Can you work these out from the model? Positions are in its coordinate system, mm. Face numbers are marked on the shaded views. A direction names the side the tool comes from. Give positions to 0.01 mm unless a question says otherwise; leave off trailing zeros. Loops run counter-clockwise (first coordinate to the right, second up) from the corner with the lowest first, then second, coordinate; pieces in that order, holes last.
Autodesk Inventor part; units mm, degrees
ref_plane "YZ Plane" through (0, 0, 0) normal (1, 0, 0) x (0, 1, 0)
ref_plane "XZ Plane" through (0, 0, 0) normal (0, 1, 0) x (-1, 0, 0)
ref_plane "XY Plane" through (0, 0, 0) normal (0, 0, 1) x (1, 0, 0)
sketch "Sketch1" plane through (0, 0, 0) normal (0, 1, 0) x (-1, 0, 0)
  line L0 (-48.611, 110.4452) -> (-48.611, 10.4452)
  line L1 (-48.611, 111.4452) -> (52.389, 111.4452)
  line L2 (52.389, 111.4452) -> (52.389, 9.4452)
  line L3 (52.389, 9.4452) -> (-48.611, 9.4452)
  line L4 (-48.611, 10.4452) -> (-48.611, 9.4452)
  line L5 (-48.611, 110.4452) -> (-48.611, 111.4452)
  line L6 (54.389, 7.4452) -> (54.389, 113.4452)
  line L7 (54.389, 113.4452) -> (-50.611, 113.4452)
  line L8 (-50.611, 113.4452) -> (-50.611, 110.4452)
  line L9 (-50.611, 110.4452) -> (-50.611, 10.4452)
  line L10 (-50.611, 10.4452) -> (-50.611, 7.4452)
  line L11 (-50.611, 7.4452) -> (54.389, 7.4452)
  point P0 (0, 0)
  dimension "d1" = 2
extrude "Extrusion1" add sketch "Sketch1" along normal blind 25
sketch "Sketch2" plane through (0, 25, 0) normal (0, 1, 0) x (1, 0, 0)
  line L0 (-54.389, -7.4452) -> (-54.389, -113.4452)
  line L1 (50.611, -113.4452) -> (50.611, -7.4452)
  line L2 (-54.389, -113.4452) -> (50.611, -113.4452)
  line L3 (50.611, -113.4452) -> (50.611, -7.4452)
  line L4 (50.611, -7.4452) -> (-54.389, -7.4452)
  line L5 (-54.389, -7.4452) -> (-54.389, -113.4452)
  point P0 (0, 0)
extrude "Extrusion2" add sketch "Sketch2" along normal blind 2
sketch "Sketch3" plane through (0, 25, 0) normal (0, -1, 0) x (1, 0, 0)
  line L0 (48.611, 9.4452) -> (48.611, 111.4452)
  line L1 (48.611, 111.4452) -> (-52.389, 111.4452)
  line L2 (-52.389, 111.4452) -> (-52.389, 9.4452)
  line L3 (-52.389, 9.4452) -> (48.611, 9.4452)
  line L4 (-52.389, 9.4452) -> (-43.389, 9.4452)
  line L5 (-43.389, 9.4452) -> (-43.389, 18.4452)
  line L6 (-43.389, 18.4452) -> (-52.389, 18.4452)
  line L7 (-52.389, 18.4452) -> (-52.389, 9.4452)
  line L8 (48.611, 9.4452) -> (39.611, 9.4452)
  line L9 (39.611, 9.4452) -> (39.611, 18.4452)
  line L10 (39.611, 18.4452) -> (48.611, 18.4452)
  line L11 (48.611, 18.4452) -> (48.611, 9.4452)
  line L12 (48.611, 111.4452) -> (39.611, 111.4452)
  line L13 (39.611, 111.4452) -> (39.611, 102.4452)
  line L14 (39.611, 102.4452) -> (48.611, 102.4452)
  line L15 (48.611, 102.4452) -> (48.611, 111.4452)
  line L16 (-52.389, 111.4452) -> (-43.389, 111.4452)
  line L17 (-43.389, 111.4452) -> (-43.389, 102.4452)
  line L18 (-43.389, 102.4452) -> (-52.389, 102.4452)
  line L19 (-52.389, 102.4452) -> (-52.389, 111.4452)
  point P0 (0, 0)
  dimension "d6" = 9
  dimension "d7" = 9
  dimension "d8" = 9
  dimension "d9" = 9
  dimension "d10" = 9
  dimension "d11" = 9
  dimension "d12" = 9
extrude "Extrusion3" add sketch "Sketch3" along normal blind 23.394 contours L3 L9 L10 L0 | L14 L13 L1 L0 | L3 L2 L6 L5 | L17 L18 L2 L1
sketch "Sketch4" plane through (0, 1.606, 0) normal (0, -1, 0) x (1, 0, 0)
  line L0 (-52.389, 9.4452) -> (-52.389, 18.4452)
  line L1 (-43.389, 9.4452) -> (-52.389, 9.4452)
  line L2 (-43.389, 9.4452) -> (-43.389, 18.4452)
  line L3 (-43.389, 18.4452) -> (-52.389, 18.4452)
  line L4 (-43.389, 102.4452) -> (-43.389, 111.4452)
  line L5 (-52.389, 111.4452) -> (-43.389, 111.4452)
  line L6 (-52.389, 102.4452) -> (-52.389, 111.4452)
  line L7 (-52.389, 102.4452) -> (-43.389, 102.4452)
  line L8 (48.611, 111.4452) -> (48.611, 102.4452)
  line L9 (39.611, 111.4452) -> (48.611, 111.4452)
  line L10 (39.611, 111.4452) -> (39.611, 102.4452)
  line L11 (39.611, 102.4452) -> (48.611, 102.4452)
  line L12 (39.611, 18.4452) -> (39.611, 9.4452)
  line L13 (48.611, 9.4452) -> (39.611, 9.4452)
  line L14 (48.611, 18.4452) -> (48.611, 9.4452)
  line L15 (48.611, 18.4452) -> (39.611, 18.4452)
  line L16 (-52.389, 102.4452) -> (-52.389, 18.4452)
  line L17 (39.611, 9.4452) -> (39.611, 18.4452)
  circle A0 centre (-47.889, 13.9452) radius 1.5
  circle A1 centre (-47.889, 106.9452) radius 1.5
  circle A2 centre (44.111, 106.9452) radius 1.5
  circle A3 centre (44.111, 13.9452) radius 1.5
  point P0 (0, 0)
  dimension "d15" = 3
  dimension "d16" = 3
  dimension "d17" = 3
  dimension "d18" = 3
extrude "Extrusion4" cut sketch "Sketch4" against normal blind 20 contours A0 | A1 | A2 | A3
sketch "Sketch5" plane through (50.611, 0, 113.4452) normal (1, 0, 0) x (0, 0, -1)
  line L0 (71.0695, 1.15) -> (65.3163, 1.15)
  line L1 (71.0695, 8.15) -> (65.3163, 8.15)
  arc A0 (65.3163, 8.15) -> (65.3163, 1.15) centre (65.3163, 4.65) ccw
  arc A1 (71.0695, 1.15) -> (71.0695, 8.15) centre (71.0695, 4.65) ccw
  line L2 (106, 0) -> (0, 0)
  point P0 (113.4452, 0)
extrude "Extrusion5" cut sketch "Sketch5" against normal blind 20
sketch "Sketch6" plane through (0, 27, 0) normal (0, 1, 0) x (1, 0, 0)
  line L0 (37.644, -52.7652) -> (37.644, -53.7652)
  line L1 (41.578, -53.7652) -> (41.578, -52.7652)
  line L2 (37.644, -53.7652) -> (41.578, -53.7652)
  line L3 (41.578, -53.7652) -> (41.578, -52.7652)
  line L4 (41.578, -52.7652) -> (37.644, -52.7652)
  line L5 (37.644, -52.7652) -> (37.644, -53.7652)
  point P0 (0, 0)
extrude "Extrusion6" cut sketch "Sketch6" against normal blind 20
sketch "Sketch7" plane through (0, 27, 0) normal (0, 1, 0) x (1, 0, 0)
  circle A0 centre (-24.1564, -107.1543) radius 1.9651
  circle A1 centre (-38.523, -70.7508) radius 1.9118
  circle A2 centre (42.3862, -71.3336) radius 1.8923
  line L0 (32.644, -52.7652) -> (32.644, -53.7652)
  line L1 (36.578, -53.7652) -> (36.578, -52.7652)
  line L2 (32.644, -53.7652) -> (36.578, -53.7652)
  line L3 (36.578, -53.7652) -> (36.578, -52.7652)
  line L4 (36.578, -52.7652) -> (32.644, -52.7652)
  line L5 (32.644, -52.7652) -> (32.644, -53.7652)
  point P0 (0, 0)
extrude "Extrusion7" cut sketch "Sketch7" against normal blind 2
sketch "Sketch8" plane through (0, 27, 0) normal (0, 1, 0) x (1, 0, 0)
  circle A0 centre (42.3862, -71.3336) radius 1.8923
  circle A1 centre (-24.1564, -107.1543) radius 1.9651
  line L0 (32.644, -52.7652) -> (36.578, -52.7652)
  line L1 (36.578, -52.7652) -> (36.578, -53.7652)
  line L2 (36.578, -53.7652) -> (32.644, -53.7652)
  line L3 (32.644, -53.7652) -> (32.644, -52.7652)
  circle A2 centre (-38.523, -70.7508) radius 1.9118
  line L4 (37.644, -52.7652) -> (41.578, -52.7652)
  line L5 (41.578, -52.7652) -> (41.578, -53.7652)
  line L6 (41.578, -53.7652) -> (37.644, -53.7652)
  line L7 (37.644, -53.7652) -> (37.644, -52.7652)
  line L8 (50.611, -113.4452) -> (50.611, -7.4452)
  line L9 (50.611, -7.4452) -> (-54.389, -7.4452)
  line L10 (-54.389, -7.4452) -> (-54.389, -113.4452)
  line L11 (-54.389, -113.4452) -> (50.611, -113.4452)
  line L12 (-54.389, -113.4452) -> (50.611, -113.4452)
  arc A3 (-2.7981, -50.4866) -> (-0.7981, -50.5048) centre (-1.889, -60.4452) ccw
  line L13 (-2.7981, -50.4866) -> (-2.7981, -49.4866)
  line L14 (-2.7981, -49.4866) -> (-0.7981, -49.4866)
  line L15 (-0.7981, -49.4866) -> (-0.7981, -50.5048)
  point P0 (0, 0)
  dimension "d37" = 1
  dimension "d38" = 2
extrude "Extrusion8" cut sketch "Sketch8" against normal blind 2 contours L13 L14 L15 A3
properties part number "Parte inferior"
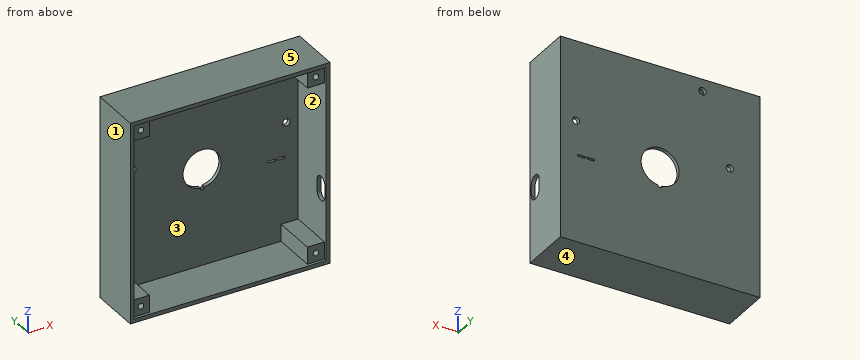
(1) Suppose I cut it at C-C on y = 9.5. List the corners of the cut face in (x, z) for me, plus the area to 3 significant figures.
Returned:
outline: (-54.39, 7.45) - (50.61, 7.45) - (50.61, 113.45) - (-54.39, 113.45) - close; hole (-52.39, 18.45) - (-43.39, 18.45) - (-43.39, 9.45) - (39.61, 9.45) - (39.61, 18.45) - (48.61, 18.45) - (48.61, 102.45) - (39.61, 102.45) - (39.61, 111.45) - (-43.39, 111.45) - (-43.39, 102.45) - (-52.39, 102.45) - close; hole circle Ø3 at (-47.89, 13.95); hole circle Ø3 at (-47.89, 106.95); hole circle Ø3 at (44.11, 13.95); hole circle Ø3 at (44.11, 106.95)
area: 1,120 mm2
(2) Will these pins go through, and if not, where does the flat tip stop? P1, Ø3, axis at x = -28.5, z = 58, coming from the -Y side; P2, Ø2.5, axis at x = 43.5, z = 14, coming from the -Y side; P3, Ø2.5, axis at x = 44, z = 14, coming from the -Y side.
Returned:
P1: stops at y = 25
P2: stops at y = 1.61
P3: stops at y = 21.61
(3) Which directions (+Z, -Z, +X, -X, +Y, -Y) give clear straight access to the entire face, cutting with the end or side of a thin tool? Please do the marked faces 1 and 2.
Returned:
face 1: +Z, -Z, -X, +Y, -Y
face 2: -Y
(4) Suppose I cut it at A-A on x = 35. List the corners of the cut face in (y, z) for me, plus the area to 3 significant figures.
Returned:
outline: (0, 7.45) - (27, 7.45) - (27, 52.77) - (25, 52.77) - (25, 9.45) - (0, 9.45) - close; (0, 111.45) - (25, 111.45) - (25, 53.77) - (27, 53.77) - (27, 113.45) - (0, 113.45) - close
area: 310 mm2
(5) Please list where these lines run through material, in increasing order: probe 1 along Z at (x, y) = (15.5, 16.25); probe 2 along X at (y, z) = (22.5, 103); probe 3 along X at (y, z) = (7.5, 14).
Returned:
probe 1: z = 7.45 to 9.45, 111.45 to 113.45
probe 2: x = -54.39 to -43.39, 39.61 to 50.61
probe 3: x = -54.39 to -49.39, -46.39 to -43.39, 39.61 to 42.61, 45.61 to 50.61
(6) Thinking about a two-plate mould opening in Z: for the marked faces 3, 4 and 5, which applies, pulls with the +Z half, pulls with the -Z half, needs draft (parallel to the pull), parting line crosses it, or undercut?
Returned:
face 3: undercut
face 4: pulls with the -Z half
face 5: pulls with the +Z half
(7) Suppose I cut it at D-D on z = 100. List the corners of the cut face in (x, y) for me.
Returned:
outline: (-54.39, 0) - (-52.39, 0) - (-52.39, 25) - (48.61, 25) - (48.61, 0) - (50.61, 0) - (50.61, 27) - (-54.39, 27) - close
(8) Suppose I cut it at B-B on z = 59. List the corners of the cut face in (x, y) for me, plus the area to 3 significant figures.
Returned:
outline: (-54.39, 0) - (-52.39, 0) - (-52.39, 25) - (-11.78, 25) - (-11.78, 27) - (-54.39, 27) - close; (8.01, 25) - (48.61, 25) - (48.61, 0) - (50.61, 0) - (50.61, 27) - (8.01, 27) - close
area: 270 mm2
